Source: CAD feature listing. Evaluate the final solid. Frame: model axes, mm. A direction names the side the tool comes from. Round coordinates to 2 decimals unless told otherwise and drop trailing zeros. Order: outer loops, then holes, each group sorted by start corner. A loop starts at its lowest first (then second) coordinate and runs counter-clockwise, first axis right, second up. Notation, with made-up numbers: (-5.75, 4.25) -> (29.25, 4.25) arc R12 ccw to (29.25, 24.25) -> close; hole circle Ø5 at (53.5, 77.25). An arc over 180 degrees is marked (long way). Write item = value, one per line. Start each with the question number.
(1) Contact query for flat-ended pins moving along their axis: pin 1 Ø1.5 at (x, y) = (-4, 5.5) entering from +Z; pin 2 Ø5 at (x, y) = (4, 5) entering from -Z. Output: stop coordinate, or through.
(2) Draft query along Z for faces 1 (the face through (-9.5, 5, 0)), 2 (the face through (-0.998, 0.74, -1.245)), 3 (the face through (-2, 5, -9.5)). Return one class per face: released by +Z, released by -Z, zero draft, split by the parting line, or undercut.
(3) Cut plane B-B on x = 4. Return the cut outline in (y, z) (3 decimals).
(4) Cut plane A-A on y = 5. Return the cut outline in (x, z) (3 decimals).
(5) Cut plane D-D on z = 7. Return the cut outline in (x, y) (3 decimals).
(6) Ray query, line 1 (Z direction, x = -4, y = 1.1); line 2 (Z direction, x = 4, y = 1.4); line 3 (X direction, y = 7.25, z = 0). Return the intervals inside material, ascending.
(7) Reachability of faces 4 (the face through (0, 0, 0)), 5 (the face through (-4, 5, 4.5)), 6 (the face through (5.386, 1.085, 0.575)) from +Z, -Z, +X, -X, +Y, -Y: full face, straight path, thin tool, end or side. Return the list, or none.
(8) Cut plane C-C on z = -6.75. Return the cut outline in (x, y) (3 decimals), then the cut area to 3 significant figures.
from build123d import *

# Parameters (mm, degrees)
SKETCH2_W           = 19
SKETCH2_H           = 19
SKETCH2_R           = 3
BOSS_EXTRUDE1_DEPTH = 10
SKETCH3_R           = 3.25
CUT_EXTRUDE1_DEPTH  = 1.5
SKETCH7_R           = 3.175
CUT_EXTRUDE5_DEPTH  = 20
CUT_EXTRUDE9_REACH  = 12
SKETCH12_R          = 1.5
SKETCH14_R          = 1.5
CUT_EXTRUDE11_DEPTH = 5
CHAMFER1_SIZE       = 0.5


with BuildPart() as part:
    # Sketch2 → Boss-Extrude1 (new body)
    with BuildSketch(Plane(origin=(0, 0, 0), x_dir=(1, 0, 0), z_dir=(0, 1, 0))):
        Rectangle(SKETCH2_W, SKETCH2_H)
        with Locations((-4, 0)):
            Circle(SKETCH2_R, mode=Mode.SUBTRACT)
    extrude(amount=BOSS_EXTRUDE1_DEPTH)

    # Sketch3 → Cut-Extrude1 (cut)
    with BuildSketch(Plane.XZ):
        with Locations((-4, 0)):
            Circle(SKETCH3_R)
    extrude(amount=-CUT_EXTRUDE1_DEPTH, mode=Mode.SUBTRACT)

    # Sketch7 → Cut-Extrude5 (cut, through all)
    with BuildSketch(Plane(origin=(0, 0, -9.5), x_dir=(-1, 0, 0), z_dir=(0, 0, -1))):
        with Locations((-4, 5)):
            Circle(SKETCH7_R)
    extrude(amount=-CUT_EXTRUDE5_DEPTH, mode=Mode.SUBTRACT)

    # Sketch12 → Cut-Extrude9 (cut, up to next)
    with BuildSketch(Plane(origin=(0, 0, 0), x_dir=(1, 0, 0), z_dir=(0, 1, 0)), mode=Mode.PRIVATE) as cut_extrude9_sk1:
        with Locations((4, 0)):
            Circle(SKETCH12_R)
    cut_extrude9_tool1 = extrude(cut_extrude9_sk1.sketch, amount=CUT_EXTRUDE9_REACH, mode=Mode.PRIVATE) & part.part
    add(cut_extrude9_tool1.solids().sort_by_distance((4, 0, 0))[0], mode=Mode.SUBTRACT)

    # Sketch14 → Cut-Extrude11 (cut)
    with BuildSketch(Plane(origin=(0, 0, 9.5), x_dir=(-1, 0, 0), z_dir=(0, 0, -1))):
        with Locations((4, 5)):
            Circle(SKETCH14_R)
    extrude(amount=CUT_EXTRUDE11_DEPTH, mode=Mode.SUBTRACT)

    # Chamfer1
    chamfer1_edges = [part.edges().sort_by_distance(p)[0] for p in [
        (-9.5, 10, 0),
        (0, 10, 9.5),
        (9.5, 10, 0),
        (0, 0, 9.5),
        (-9.5, 0, 0),
        (0, 0, -9.5),
        (9.5, 0, 0),
        (0, 10, -9.5),
        (9.5, 5, 9.5),
        (-9.5, 5, 9.5),
        (-9.5, 5, -9.5),
        (9.5, 5, -9.5),
    ]]
    chamfer(chamfer1_edges, length=CHAMFER1_SIZE)


solid = part.part
Evaluation:
q1.pin_1 = 4.5
q1.pin_2 = through
q2.face_1 = zero draft
q2.face_2 = undercut
q2.face_3 = released by -Z
q3.outline = (0, -9) -> (0.5, -9.5) -> (1.825, -9.5) -> (1.825, -1.5) -> (0, -1.5) -> close; (0, 1.5) -> (1.825, 1.5) -> (1.825, 9.5) -> (0.5, 9.5) -> (0, 9) -> close; (8.175, -9.5) -> (9.5, -9.5) -> (10, -9) -> (10, 9) -> (9.5, 9.5) -> (8.175, 9.5) -> close
q4.outline = (-9.5, -9) -> (-9, -9.5) -> (0.825, -9.5) -> (0.825, 9.5) -> (-2.5, 9.5) -> (-2.5, 4.5) -> (-5.5, 4.5) -> (-5.5, 9.5) -> (-9, 9.5) -> (-9.5, 9) -> close; (7.175, -9.5) -> (9, -9.5) -> (9.5, -9) -> (9.5, 9) -> (9, 9.5) -> (7.175, 9.5) -> close; hole circle Ø6 at (-4, 0)
q5.outline = (-9.5, 0.5) -> (-9, 0) -> (9, 0) -> (9.5, 0.5) -> (9.5, 9.5) -> (9, 10) -> (-9, 10) -> (-9.5, 9.5) -> close; hole circle Ø3 at (-4, 5); hole circle Ø6.35 at (4, 5)
q6.line_1 = -9.5 to -3.25, 3.25 to 9.5
q6.line_2 = -9.5 to -1.5, 1.5 to 9.5
q6.line_3 = -9.5 to -7, -1 to 1.76, 6.24 to 9.5
q7.face_4 = +Z, -Z, +X, -X, -Y
q7.face_5 = +Z
q7.face_6 = -Y
q8.outline = (-9.5, 0.5) -> (-9, 0) -> (9, 0) -> (9.5, 0.5) -> (9.5, 9.5) -> (9, 10) -> (-9, 10) -> (-9.5, 9.5) -> close; hole circle Ø6.35 at (4, 5)
q8.area = 158 mm^2
